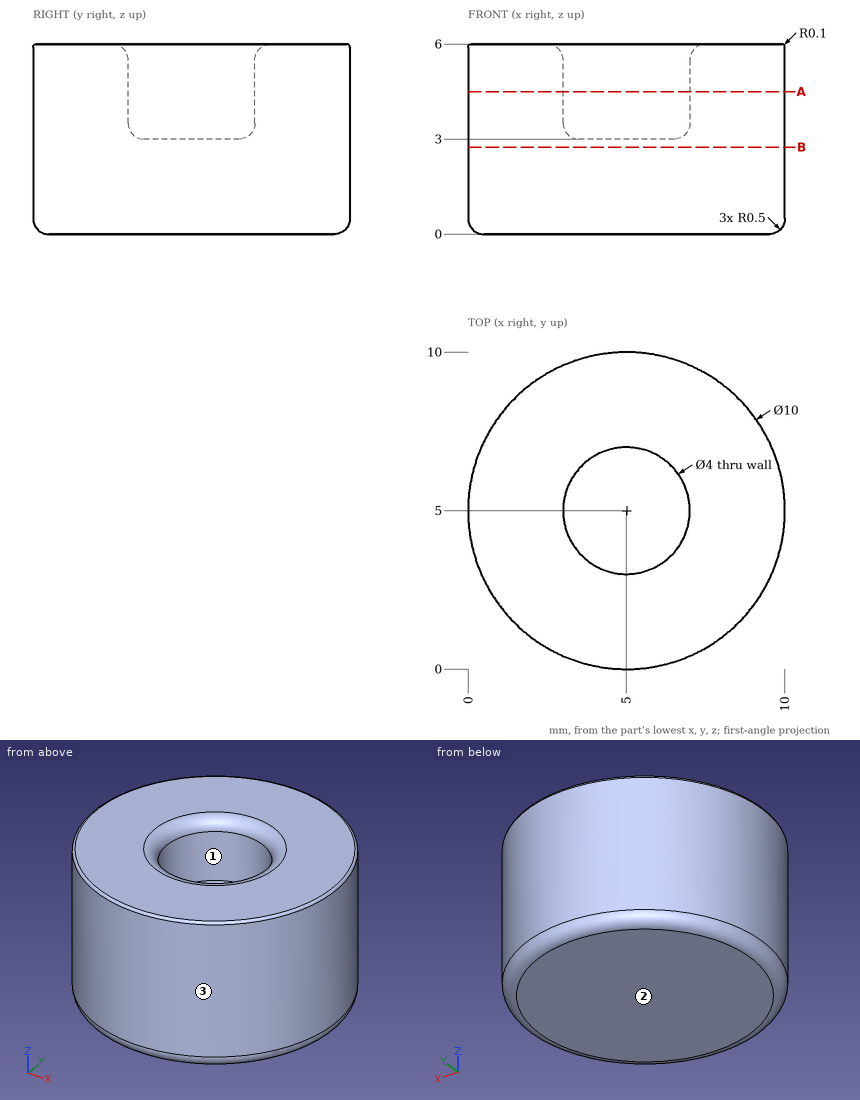
Part print with two shaded views. Sizes in mm from the minimum x, y, z corner. Round coordinates to 2 decimals unless told otherwise and drop trailing zeros. Order: outer loops, then holes, each group sorted by start corner. A loop starts at its lowest first (then second) coordinate and runs counter-clockwise, first axis right, second up. Notation, with made-up numbers: (-35, 37) -> (18, 37) arc R24 ccw to (18, 69) -> close; hole circle Ø2 at (88, 2). An arc over 180 degrees is marked (long way). Use one line per item in the form item = value.
Item 1: Drill centre lines: line 1 (Y direction, x = 5, z = 4.1); line 2 (X direction, y = 5.75, z = 4); line 3 (X direction, y = 6, z = 4.5). Where is each one in solid material? Low to high.
Returned:
line_1 = 0 to 3, 7 to 10
line_2 = 0.06 to 3.15, 6.85 to 9.94
line_3 = 0.1 to 3.27, 6.73 to 9.9
Item 2: Cut at B-B, the plane z = 2.75. Write the cut outline in (x, y).
Returned:
outline = circle Ø10 at (5, 5)
Item 3: Flat gauge pins, fed straight in: pin 1 Ø1 at (x, z) = (1.5, 4) entering from -Y; pin 2 Ø1.5 at (x, y) = (5.5, 4.5) entering from +Z; pin 3 Ø1 at (y, z) = (2.5, 4) entering from +X. Where does each tip first touch, or does it go through?
Returned:
pin_1 = 1
pin_2 = 3
pin_3 = 9.58
Item 4: Pull direction X, two halves, no side cores. Call the marked faces 1, 2 and 3: released by +X, released by -X, zero draft, split by the parting line, or undercut.
Returned:
face_1 = undercut
face_2 = zero draft
face_3 = split by the parting line
Item 5: Cut at A-A, the plane z = 4.5. Write the cut outline in (x, y).
Returned:
outline = circle Ø10 at (5, 5); hole circle Ø4 at (5, 5)
